For this review, take the finished solid that the model builds, in its own axes (mm). A direction names the side the tool comes from. Round coordinates to 2 decimals unless told otherwise and drop trailing zeros. Write each loop counter-clockwise with the first axis right and the second up, starting at its lowest first coordinate (ties: lowest second). Pieces come first, ordered by that corner, then holes. Notation, with made-up numbers: (-21.5, 21) - (35.5, 21) arc R9 ccw to (35.5, 34) - close; hole circle Ø11 at (71.5, 31). An arc over 180 degrees is marked (long way). Answer in a Markdown table with one row per item. Add a question column.
from build123d import *

# Parameters (mm, degrees)
SKETCH1_W                                       = 60
SKETCH1_H                                       = 26
BOSS_EXTRUDE1_DEPTH                             = 2
SKETCH2_W                                       = 58
SKETCH2_H                                       = 24
SKETCH2_W_2                                     = 56
SKETCH2_H_2                                     = 22
BOSS_EXTRUDE2_DEPTH                             = 3
SKETCH3_R                                       = 1.5
SKETCH3_R_2                                     = 0.75
BOSS_EXTRUDE3_DEPTH                             = 5
SKETCH6_R                                       = 2.5
BOSS_EXTRUDE4_DEPTH                             = 3
CSK_FOR_M3_FLAT_HEAD_MACHINE_SCREW1_D           = 3.4
CSK_FOR_M3_FLAT_HEAD_MACHINE_SCREW1_CSINK_D     = 6.3
CSK_FOR_M3_FLAT_HEAD_MACHINE_SCREW1_CSINK_ANGLE = 90


with BuildPart() as part:
    # Sketch1 → Boss-Extrude1 (new body)
    with BuildSketch(Plane(origin=(0, 0, 0), x_dir=(1, 0, 0), z_dir=(0, 1, 0))):
        with Locations((30, 13)):
            Rectangle(SKETCH1_W, SKETCH1_H)
    extrude(amount=BOSS_EXTRUDE1_DEPTH)

    # Sketch2 → Boss-Extrude2 (add)
    with BuildSketch(Plane(origin=(0, 2, 0), x_dir=(1, 0, 0), z_dir=(0, 1, 0))):
        with Locations((30, 13)):
            Rectangle(SKETCH2_W, SKETCH2_H)
        with Locations((30, 13)):
            Rectangle(SKETCH2_W_2, SKETCH2_H_2, mode=Mode.SUBTRACT)
    extrude(amount=BOSS_EXTRUDE2_DEPTH)

    # Sketch3 → Boss-Extrude3 (add)
    # profile 1 of 3: a face of its own
    with BuildSketch(Plane(origin=(0, 2, 0), x_dir=(1, 0, 0), z_dir=(0, 1, 0))):
        with Locations(Location((16.5, 9.5, 0), (0, 0, 90))):
            Circle(SKETCH3_R)
        with Locations(Location((16.5, 9.5, 0), (0, 0, 270))):
            Circle(SKETCH3_R_2, mode=Mode.SUBTRACT)
    # profile 2 of 3: a face of its own
    with BuildSketch(Plane(origin=(0, 2, 0), x_dir=(1, 0, 0), z_dir=(0, 1, 0))):
        with Locations(Location((30, 9.5, 0), (0, 0, 90))):
            Circle(SKETCH3_R)
        with Locations(Location((30, 9.5, 0), (0, 0, 270))):
            Circle(SKETCH3_R_2, mode=Mode.SUBTRACT)
    # profile 3 of 3: a face of its own
    with BuildSketch(Plane(origin=(0, 2, 0), x_dir=(1, 0, 0), z_dir=(0, 1, 0))):
        with Locations(Location((43.5, 9.5, 0), (0, 0, 90))):
            Circle(SKETCH3_R)
        with Locations(Location((43.5, 9.5, 0), (0, 0, 270))):
            Circle(SKETCH3_R_2, mode=Mode.SUBTRACT)
    extrude(amount=BOSS_EXTRUDE3_DEPTH)

    # Sketch6 → Boss-Extrude4 (add)
    with BuildSketch(Plane(origin=(0, 2, 0), x_dir=(1, 0, 0), z_dir=(0, 1, 0))):
        with Locations((30, 22.5)):
            Circle(SKETCH6_R)
    extrude(amount=BOSS_EXTRUDE4_DEPTH)

    # CSK for M3 Flat Head Machine Screw1 (through all)
    with Locations(Plane(origin=(0, 0, 0), x_dir=(-1, 0, 0), z_dir=(0, -1, 0))):
        with Locations((-30, 22.5)):
            CounterSinkHole(CSK_FOR_M3_FLAT_HEAD_MACHINE_SCREW1_D / 2, CSK_FOR_M3_FLAT_HEAD_MACHINE_SCREW1_CSINK_D / 2, counter_sink_angle=CSK_FOR_M3_FLAT_HEAD_MACHINE_SCREW1_CSINK_ANGLE)


solid = part.part
Q1. Tool access review of faces 1 (the face through (16.5, 2, -9.5)), 2 (the face through (1, 3, -13)), 3 (the face through (30, 3, -1)): name each direction out of +Z, -Z, +X, -X, +Y, -Y from which nothing blocks a thin tool from reaching the whole face with its end or side.
Q2. Insertion check: pin 1 Ø6 at (x, z) = (21.5, -20) entering from +Y; pin 2 Ø1.5 at (x, y) = (47, 4) entering from +Z; pin 3 Ø1.5 at (y, z) = (3, -10) entering from -X. Each pin has a flat end and moves straight along its axis. Give the tip position at first contact, or say it passes through.
Q3. Add section A-A on y = 3.25. Count the separate pieces of the cut face and the enclosed holes in it, then the cut area to 3 significant figures.
Q4. Draft analysis for pull direction Z (two halves, no side actions). For faces 4 (the face through (44.244, 4.465, -9.598)), 5 (the face through (30, 0, -13)), 6 (the face through (30, 3, -25)), 7 (the face through (16.044, 4.465, -10.095)), state which applies: released by +Z, released by -Z, zero draft, split by the parting line, or undercut.
Q5. To check wall thickness, follow probe 1 along X at (y, z) = (5.6, -9.5); probe 2 along Z at (x, y) = (6, 3.25); probe 3 along X at (y, z) = (4.25, -14.75). State the ranges of each line that lie inside material, in increasing order.
Q6. Add section D-D on x = 54. State the section outline as (y, z) points.
Q7. Add section B-B on z = -22.5. State the section outline as (x, y) points, then the cut area to 3 significant figures.
Q8. Add section C-C on x = 43.5. State the section outline as (y, z) points, then the cut area to 3 significant figures.
Answer sheet:
| question | item | result |
|---|---|---|
| 1 | face 1 | +Y |
| 1 | face 2 | +Z, -Z, -X, +Y |
| 1 | face 3 | +Z, +X, -X, +Y |
| 2 | pin 1 | stops at y = 2 |
| 2 | pin 2 | stops at z = -1 |
| 2 | pin 3 | stops at x = 1 |
| 3 | separate pieces | 4 |
| 3 | enclosed holes | 5 |
| 3 | area | 184 mm² |
| 4 | face 4 | undercut |
| 4 | face 5 | zero draft |
| 4 | face 6 | released by -Z |
| 4 | face 7 | undercut |
| 5 | probe 1 | x = 15 to 15.75, 17.25 to 18, 28.5 to 29.25, 30.75 to 31.5, 42 to 42.75, 44.25 to 45 |
| 5 | probe 2 | z = -25 to -24, -2 to -1 |
| 5 | probe 3 | x = 1 to 2, 58 to 59 |
| 6 | outline | (0, -26) - (2, -26) - (2, -25) - (5, -25) - (5, -24) - (2, -24) - (2, -2) - (5, -2) - (5, -1) - (2, -1) - (2, 0) - (0, 0) - close |
| 7 | outline | (0, 0) - (26.85, 0) - (28.3, 1.45) - (28.3, 5) - (27.5, 5) - (27.5, 2) - (2, 2) - (2, 5) - (1, 5) - (1, 2) - (0, 2) - close; (31.7, 1.45) - (33.15, 0) - (60, 0) - (60, 2) - (59, 2) - (59, 5) - (58, 5) - (58, 2) - (32.5, 2) - (32.5, 5) - (31.7, 5) - close |
| 7 | area | 122 mm² |
| 8 | outline | (0, -26) - (2, -26) - (2, -25) - (5, -25) - (5, -24) - (2, -24) - (2, -11) - (7, -11) - (7, -10.25) - (2, -10.25) - (2, -8.75) - (7, -8.75) - (7, -8) - (2, -8) - (2, -2) - (5, -2) - (5, -1) - (2, -1) - (2, 0) - (0, 0) - close |
| 8 | area | 65.5 mm² |
